```python
from build123d import *

# Parameters (mm, degrees)
SKETCH_W     = 63
SKETCH_H     = 45
PAD_DEPTH    = 2
SKETCH002_W  = 61
SKETCH002_H  = 43
PAD001_DEPTH = 4
SKETCH003_W  = 59
SKETCH003_H  = 41
POCKET_DEPTH = 2
FILLET_R     = 1
FILLET001_R  = 0.3


with BuildPart() as part:
    # Sketch → Pad (new body)
    with BuildSketch(Plane.XY):
        Rectangle(SKETCH_W, SKETCH_H)
    extrude(amount=PAD_DEPTH)

    # Sketch002 → Pad001 (join)
    with BuildSketch(Plane.XY):
        Rectangle(SKETCH002_W, SKETCH002_H)
    extrude(amount=PAD001_DEPTH)

    # Sketch003 → Pocket (cut)
    with BuildSketch(Plane.XY.offset(4)):
        Rectangle(SKETCH003_W, SKETCH003_H)
    extrude(amount=-POCKET_DEPTH, mode=Mode.SUBTRACT)

    # Fillet
    fillet_edges = [part.edges().sort_by_distance(p)[0] for p in [
        (0, -22.5, 0),
        (31.5, 0, 0),
        (-31.5, 0, 0),
        (0, 22.5, 0),
    ]]
    fillet(fillet_edges, radius=FILLET_R)

    # Fillet001
    fillet001_edges = [part.edges().sort_by_distance(p)[0] for p in [
        (30.5, 0, 4),
        (0, 21.5, 4),
        (0, -21.5, 4),
        (-30.5, 0, 4),
    ]]
    fillet(fillet001_edges, radius=FILLET001_R)


solid = part.part
```
The listing builds one solid part. Answer for the finished solid, in the listing's coordinates (mm). A direction names the side the tool comes from. Give positions to 0.01 mm unless a question says otherwise; leave off trailing zeros. Order: outer loops, then holes, each group sorted by start corner. A loop starts at its lowest first (then second) coordinate and runs counter-clockwise, first axis right, second up.
Item 1: Given pin 1 Ø1.9 at (x, z) = (-15, 3) entering from +Y; pin 2 Ø1.4 at (y, z) = (5.5, 3) entering from -X; pin 3 Ø20.5 at (x, y) = (4, 3) entering from +Z, each flat-ended and moving along its own axis, determine where each tip first touches the part or whether it passes through.
From the geometry:
pin 1: stops at y = 21.5
pin 2: stops at x = -30.5
pin 3: stops at z = 2
Item 2: For a pull along X with two mould halves and no side action, classify faces 5 (the face through (30.5, 0, 3)), 6 (the face through (0, 22, 2)), 7 (the face through (-30.5, 0, 3)), 8 (the face through (0, -20.5, 3)) as pulls with the +X half, pulls with the -X half, needs draft (parallel to the pull), parting line crosses it, or undercut.
From the geometry:
face 5: pulls with the +X half
face 6: needs draft
face 7: pulls with the -X half
face 8: undercut
Item 3: Which of the six approach directions +Z, -Z, +X, -X, +Y, -Y give full straight-line access (tool end or side, diameter ignored) to faces 1 (the face through (0, -21.5, 3)), 2 (the face through (0, 21, 4)), 3 (the face through (29.5, 0, 3)), 4 (the face through (0, 21.5, 3))?
From the geometry:
face 1: +Z, +X, -X, -Y
face 2: +Z, +X, -X, +Y, -Y
face 3: +Z
face 4: +Z, +X, -X, +Y
Item 4: The part is cut by section A-A, the plane z = 3.1. Give the vertices of the cut face in (x, y), and give its area (3 significant figures).
From the geometry:
outline: (-30.5, -21.5) - (30.5, -21.5) - (30.5, 21.5) - (-30.5, 21.5) - close; hole (-29.5, -20.5) - (29.5, -20.5) - (29.5, 20.5) - (-29.5, 20.5) - close
area: 204 mm2
Item 5: The part is cut by section B-B, the plane x = 3.5. Give the vertices of the cut face in (y, z), and give its area (3 significant figures).
From the geometry:
outline: (-22.5, 1) arc R1 ccw to (-21.5, 0) - (21.5, 0) arc R1 ccw to (22.5, 1) - (22.5, 2) - (21.5, 2) - (21.5, 3.7) arc R0.3 ccw to (21.2, 4) - (20.5, 4) - (20.5, 2) - (-20.5, 2) - (-20.5, 4) - (-21.2, 4) arc R0.3 ccw to (-21.5, 3.7) - (-21.5, 2) - (-22.5, 2) - close
area: 93.5 mm2
Item 6: Find the intervals of material crossed by probe 1 along Y at (x, z) = (-3, 3.4); probe 2 along X at (y, z) = (19.5, 3.6); probe 3 along Z at (x, y) = (28, 9), in increasing order.
From the geometry:
probe 1: y = -21.5 to -20.5, 20.5 to 21.5
probe 2: x = -30.5 to -29.5, 29.5 to 30.5
probe 3: z = 0 to 2
Item 7: The part is cut by section C-C, the plane y = -8. Give the vertices of the cut face in (x, z), and give its area (3 significant figures).
From the geometry:
outline: (-31.5, 1) arc R1 ccw to (-30.5, 0) - (30.5, 0) arc R1 ccw to (31.5, 1) - (31.5, 2) - (30.5, 2) - (30.5, 3.7) arc R0.3 ccw to (30.2, 4) - (29.5, 4) - (29.5, 2) - (-29.5, 2) - (-29.5, 4) - (-30.2, 4) arc R0.3 ccw to (-30.5, 3.7) - (-30.5, 2) - (-31.5, 2) - close
area: 130 mm2
